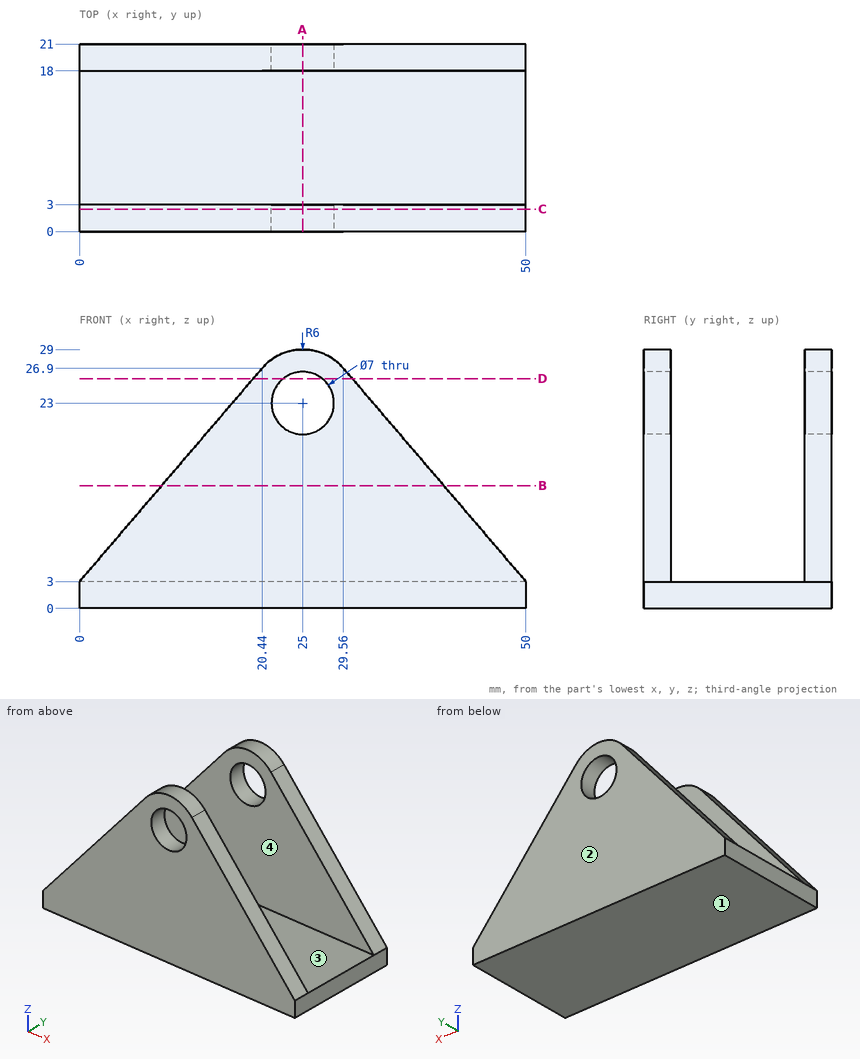
Geometry: see drawing. Coordinates: mm, zero at the bounding-box minimum. Round coordinates to 2 decimals unless told otherwise and drop trailing zeros. Write each loop counter-clockwise with the first axis right and the second up, starting at its lowest first coordinate (ties: lowest second). Pieces come first, ordered by that corner, then holes. Notation, with made-up numbers: (16.5, 79.25) -> (72.5, 79.25) arc R14 ccw to (72.5, 84.25) -> close; hole circle Ø4 at (-31, 86). An arc over 180 degrees is marked (long way). Answer as CSV lines item,"result".
1. Section C-C (y = 2.5). Return the cut outline in (x, z), plus the area to 3 significant figures.
Geometry says:
outline,"(0, 0) -> (50, 0) -> (50, 3) -> (29.56, 26.9) arc R6 ccw to (20.44, 26.9) -> (0, 3) -> close; hole circle Ø7 at (25, 23)"
area,"831 mm^2"
2. Ray query, L1, parallel to Y at x = 35, z = 15.75; L2, parallel to Z at x = 24, y = 3.75; L3, parallel to X at y = 2.05, z = 23 (1 decimal). Return the intervals inside material, ascending. Write a range as [from, to].
Geometry says:
L1,"y = [0, 3], [18, 21]"
L2,"z = [0, 3]"
L3,"x = [17.1, 21.5], [28.5, 32.9]"
3. Section A-A (x = 25). Return the cut outline in (y, z), plus the area to 3 significant figures.
Geometry says:
outline,"(0, 0) -> (21, 0) -> (21, 19.5) -> (18, 19.5) -> (18, 3) -> (3, 3) -> (3, 19.5) -> (0, 19.5) -> close; (0, 26.5) -> (3, 26.5) -> (3, 29) -> (0, 29) -> close; (18, 26.5) -> (21, 26.5) -> (21, 29) -> (18, 29) -> close"
area,"177 mm^2"
4. Section B-B (z = 13.75). Return the cut outline in (x, y), plus the area to 3 significant figures.
Geometry says:
outline,"(9.19, 0) -> (40.81, 0) -> (40.81, 3) -> (9.19, 3) -> close; (9.19, 18) -> (40.81, 18) -> (40.81, 21) -> (9.19, 21) -> close"
area,"190 mm^2"
5. Contact query for flat-ended pins moving along their axis: P1, Ø6, axis at x = 40.5, y = 10.5, coming from the -Z side; P2, Ø12, axis at x = 30.5, y = 11, coming from the +Z side. Output: stop coordinate, or through.
Geometry says:
P1,"stops at z = 0"
P2,"stops at z = 3"
6. Section D-D (z = 25.75). Return the cut outline in (x, y) (1 decimal).
Geometry says:
outline,"(19.5, 0) -> (22.8, 0) -> (22.8, 3) -> (19.5, 3) -> close; (19.5, 18) -> (22.8, 18) -> (22.8, 21) -> (19.5, 21) -> close; (27.2, 0) -> (30.5, 0) -> (30.5, 3) -> (27.2, 3) -> close; (27.2, 18) -> (30.5, 18) -> (30.5, 21) -> (27.2, 21) -> close"
7. Mould query, pull axis Y, two halves, no side actions, for the marked faces 1, 2, 3 and 4. Classes: +Y half, -Y half, draft (parallel to the pull), parting line (faces both ways), or undercut.
Geometry says:
face 1,"draft"
face 2,"+Y half"
face 3,"undercut"
face 4,"undercut"
